Autodesk Inventor part; units mm, degrees
ref_plane "YZ Plane" through (0, 0, 0) normal (1, 0, 0) x (0, 1, 0)
ref_plane "XZ Plane" through (0, 0, 0) normal (0, 1, 0) x (-1, 0, 0)
ref_plane "XY Plane" through (0, 0, 0) normal (0, 0, 1) x (1, 0, 0)
sketch "Sketch2" plane through (0, 0, 0) normal (0, 1, 0) x (-1, 0, 0)
  line L0 (-23.5, 10) -> (23.5, 10)
  line L1 (23.5, 10) -> (23.5, -10)
  line L2 (23.5, -10) -> (17.5, -10)
  line L3 (-23.5, -10) -> (-23.5, 10)
  line L4 (-23.5, 10) -> (23.5, -10) construction
  line L5 (23.5, 10) -> (-23.5, -10) construction
  line L6 (21.5, 16) -> (11.5, 16)
  line L7 (11.5, 16) -> (11.5, 10)
  line L8 (11.5, 10) -> (21.5, 10)
  line L9 (21.5, 10) -> (21.5, 16)
  line L10 (-23.5, -10) -> (23.5, -77.123)
  line L11 (-23.5, -10) -> (58.442, -10) construction
  line L12 (23.5, -77.123) -> (23.5, -10)
  line L13 (20.6321, -73.0272) -> (13.7492, -63.1974)
  line L14 (13.7492, -63.1974) -> (8.8343, -66.6388)
  line L15 (8.8343, -66.6388) -> (15.7172, -76.4687)
  line L16 (15.7172, -76.4687) -> (20.6321, -73.0272)
  line L17 (6.8663, -53.3675) -> (-0.0166, -43.5377)
  line L18 (1.9514, -56.809) -> (6.8663, -53.3675)
  line L19 (-4.9315, -46.9792) -> (1.9514, -56.809)
  line L20 (-0.0166, -43.5377) -> (-4.9315, -46.9792)
  line L21 (-6.8996, -33.7079) -> (-13.7825, -23.8781)
  line L22 (-11.8145, -37.1494) -> (-6.8996, -33.7079)
  line L23 (-18.6974, -27.3195) -> (-11.8145, -37.1494)
  line L24 (-13.7825, -23.8781) -> (-18.6974, -27.3195)
  line L25 (1.5, 10) -> (-8.5, 10)
  line L26 (-8.5, 10) -> (-8.5, 16)
  line L27 (-8.5, 16) -> (1.5, 16)
  line L28 (1.5, 16) -> (1.5, 10)
  line L29 (-19.5182, -15.6866) -> (-23.5, -10)
  line L30 (-23.5, -10) -> (-28.4149, -13.4415)
  line L31 (-28.4149, -13.4415) -> (-24.4331, -19.128)
  line L32 (-24.4331, -19.128) -> (-19.5182, -15.6866)
  line L33 (17.5, -50.8098) -> (12.4, -50.8098)
  line L34 (12.4, -50.8098) -> (12.4, -41.1098)
  line L35 (12.4, -41.1098) -> (17.5, -41.1098)
  line L36 (17.5, -41.1098) -> (17.5, -50.8098)
  line L37 (17.5, -30.8098) -> (12.4, -30.8098)
  line L38 (17.5, -21.1098) -> (17.5, -30.8098)
  line L39 (12.4, -21.1098) -> (17.5, -21.1098)
  line L40 (12.4, -30.8098) -> (12.4, -21.1098)
  line L41 (17.5, -10.8098) -> (12.4, -10.8098)
  line L42 (17.5, -1.1098) -> (17.5, -10.8098)
  line L43 (12.4, -1.1098) -> (17.5, -1.1098)
  line L44 (12.4, -10.8098) -> (12.4, -1.1098)
  line L45 (12.4, -10) -> (-23.5, -10)
  line L46 (17.5, -10) -> (12.4, -10)
  point P0 (0, 0)
  dimension "d9" = 20
  dimension "d19" = 10
  dimension "d20" = 6
  dimension "d21" = 2
  dimension "d41" = 55
  dimension "d42" = 6
  dimension "d45" = 24
  dimension "d50" = 5
  dimension "d51" = 12
  dimension "d52" = 10
  dimension "d53" = 6
  dimension "d54" = 10
  dimension "d55" = 47
  dimension "d56" = 10
  dimension "d57" = 5.1
  dimension "d58" = 9.7
  dimension "d61" = 20
  dimension "d66" = 6
  dimension "d67" = 6
extrude "Extrusion2" add sketch "Sketch2" along normal blind 6 contours L0 L1 L2 L42 L43 L44 L45 L3 | L26 L27 L28 L0 | L45 L44 L41 L42 L2 L12 L10 | L7 L6 L9 L0 | L10 L22 L23 L24 | L10 L18 L19 L20 | L16 L15 L14 L10
properties part number "phone_holder_slider_side" material "Acrylic, Clear"
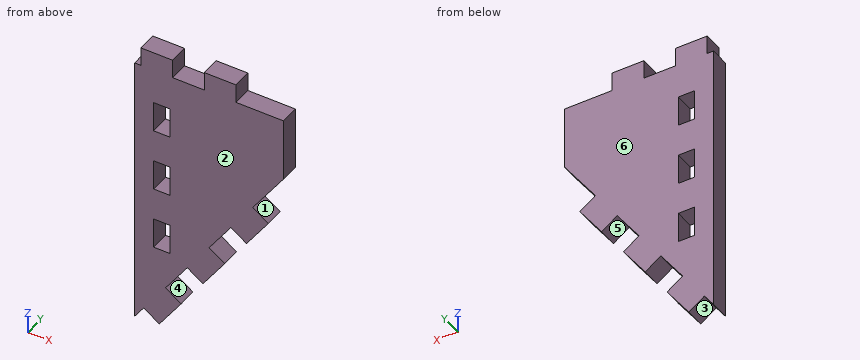
Model file for the job. Use its own axes, mm. Face numbers are marked on the shaded views. A direction names the side the tool comes from. Give positions to 0.01 mm unless a question says otherwise; leave off trailing zeros. Write each loop counter-clockwise with the first axis right and the second up, starting at its lowest first coordinate (ties: lowest second). Pieces come first, ordered by that corner, then holes. Notation, with made-up numbers: M 27,71 L 79,71 A22 ccw 79,100 Z; hole C 88,74.25 d10. An arc over 180 degrees is marked long. One line per item, written item: value. Start each with the question number.
Q1. Saw through at D-D, the plane x = -5. Write the cut outline in (y, z), plus the area to 3 significant figures.
Q2. Saw through at B-B, the plane z = -26. Write the cut outline in (x, y).
Q3. Two-plate mould, pull along X, no slides. Class the marked faces 1, 2 and 3: +X half, -X half, draft (parallel to the pull), parting line (faces both ways), or undercut.
Q4. Saw through at C-C, the plane y = 3.75. State how many separate pieces and enclosed holes the cut face has, plus the area to 3 significant figures.
Q5. Probe probe 1 along Z at (x, y) = (-15, 3.5); probe 2 along X at (y, z) = (0.3, 11); probe 3 along X at (y, z) = (4.15, -60). List the from-to ranges inside material, lowest first. Write a range as [from, to].
Q6. 3-axis set-ups, long thin cutter, end or side, ignore diameter. For the marked faces 4, 5 and 6: which of +Z, -Z, +X, -X, +Y, -Y reach the whole face in a straight line?
Q7. Saw through at A-A, the plane z = -6. Write the cut outline in (x, y).
Q8. Drop flat-ended pins along their axis: pin 1 Ø1.6 at (x, y) = (-22, 4.5) entering from +Z; pin 2 Ø1.8 at (y, z) = (2.5, 12.5) entering from +X; pin 3 Ø3 at (x, y) = (16, 2.5) entering from +Z; pin 4 Ø2.5 at (x, y) = (-14.5, 4) entering from -Z. Give the stop position or say it passes through.
Output values:
1. outline: M 0,-54.67 L 6,-54.67 L 6,10 L 0,10 Z
1. area: 388 mm²
2. outline: M -23.5,0 L -17.5,0 L -17.5,6 L -23.5,6 Z; M -12.4,0 L 16.81,0 L 16.81,6 L -12.4,6 Z
3. face 1: +X half
3. face 2: draft
3. face 3: undercut
4. separate pieces: 1
4. enclosed holes: 3
4. area: 2,700 mm²
5. probe 1: z = [-75.44, -50.81], [-41.11, -30.81], [-21.11, -10.81], [-1.11, 16]
5. probe 2: x = [-21.5, -11.5], [-1.5, 8.5]
5. probe 3: x = [-23.5, -11.51]
6. face 4: +X, +Y, -Y
6. face 5: -Z, +Y, -Y
6. face 6: +Z, -Z, +X, -X, +Y
7. outline: M -23.5,0 L -17.5,0 L -17.5,6 L -23.5,6 Z; M -12.4,0 L 23.5,0 L 23.5,6 L -12.4,6 Z
8. pin 1: stops at z = 16
8. pin 2: stops at x = 8.5
8. pin 3: stops at z = 10
8. pin 4: stops at z = -76.47
